from build123d import *

# Parameters (mm, degrees)
SKETCH1_W                      = 53
SKETCH1_H                      = 25
SKETCH1_R                      = 4.5
SKETCH1_R_2                    = 1.5
BASE_FLANGE1_DEPTH             = 1
EDGE_FLANGE1_STRIP_W           = 5.4732
EDGE_FLANGE1_STRIP_H           = 1
EDGE_FLANGE1_STRIP_CUT_DEPTH   = 25
EDGE_FLANGE1_STRIP_2_W         = 5.4732
EDGE_FLANGE1_STRIP_2_H         = 1
EDGE_FLANGE1_STRIP_CUT_2_DEPTH = 25
EDGE_FLANGE1_DEPTH             = 25
EDGE_FLANGE1_BEND_DEPTH        = 25
CUT_EXTRUDE1_DEPTH             = 73.584433593
CUT_EXTRUDE1_DEPTH_BACK        = 73.584433593
SKETCH13_R                     = 4.5
SKETCH13_R_2                   = 2
SKETCH13_R_3                   = 1.5
FILLET1_R                      = 12.5


# Sheet-metal steps are written as plain solids
with BuildPart() as part:
    # Sketch1 → Base-Flange1 (new body)
    with BuildSketch(Plane(origin=(0, 0, 0), x_dir=(1, 0, 0), z_dir=(0, 1, 0))):
        Rectangle(SKETCH1_W, SKETCH1_H)
        with Locations(Location((0, 0, 0), (0, 0, 270))):
            Circle(SKETCH1_R, mode=Mode.SUBTRACT)
        with Locations(Location((-7, 0, 0), (0, 0, 270))):
            Circle(SKETCH1_R_2, mode=Mode.SUBTRACT)
        with Locations(Location((7, 0, 0), (0, 0, 270))):
            Circle(SKETCH1_R_2, mode=Mode.SUBTRACT)
        with Locations(Location((0, 7, 0), (0, 0, 270))):
            Circle(SKETCH1_R_2, mode=Mode.SUBTRACT)
        with Locations(Location((0, -7, 0), (0, 0, 270))):
            Circle(SKETCH1_R_2, mode=Mode.SUBTRACT)
    extrude(amount=BASE_FLANGE1_DEPTH)

    # Edge-Flange1 strip (across the edge) → Edge-Flange1 strip cut (cut)
    with BuildSketch(Plane(origin=(-26.5, 1, -12.5), x_dir=(1, 0, 0), z_dir=(0, 0, 1))):
        with Locations((-2, -0.5)):
            Rectangle(EDGE_FLANGE1_STRIP_W, EDGE_FLANGE1_STRIP_H)
    extrude(amount=EDGE_FLANGE1_STRIP_CUT_DEPTH, mode=Mode.SUBTRACT)

    # Edge-Flange1 strip 2 (across the edge) → Edge-Flange1 strip cut 2 (cut)
    with BuildSketch(Plane(origin=(26.5, 1, 12.5), x_dir=(-1, 0, 0), z_dir=(0, 0, -1))):
        with Locations((-2, -0.5)):
            Rectangle(EDGE_FLANGE1_STRIP_2_W, EDGE_FLANGE1_STRIP_2_H)
    extrude(amount=EDGE_FLANGE1_STRIP_CUT_2_DEPTH, mode=Mode.SUBTRACT)

    # Edge-Flange1 section (across the edge) → Edge-Flange1 (add)
    with BuildSketch(Plane(origin=(-26.5, 1, -12.5), x_dir=(1, 0, 0), z_dir=(0, 0, 1))):
        with BuildLine():
            Line((-1, 0.7366), (-1, 65))
            Line((-1, 65), (0, 65))
            Line((0, 65), (0, 0.7366))
            ThreePointArc((0, 0.7366), (0.215745145, 0.215745145), (0.7366, 0))
            Line((0.7366, 0), (0.7366, -1))
            ThreePointArc((0.7366, -1), (-0.491361636, -0.491361636), (-1, 0.7366))
        make_face()
    extrude(amount=EDGE_FLANGE1_DEPTH)

    # Edge-Flange1 section 2 (across the edge) → Edge-Flange1 bend (add)
    with BuildSketch(Plane(origin=(26.5, 1, 12.5), x_dir=(-1, 0, 0), z_dir=(0, 0, -1))):
        with BuildLine():
            Line((-1, 0.7366), (-1, 65))
            Line((-1, 65), (0, 65))
            Line((0, 65), (0, 0.7366))
            ThreePointArc((0, 0.7366), (0.215745145, 0.215745145), (0.7366, 0))
            Line((0.7366, 0), (0.7366, -1))
            ThreePointArc((0.7366, -1), (-0.491361636, -0.491361636), (-1, 0.7366))
        make_face()
    extrude(amount=EDGE_FLANGE1_BEND_DEPTH)

    # Sketch13 → Cut-Extrude1 (cut, two sides: drawn at the far end of the back side and taken through both)
    with BuildSketch(Plane(origin=(0, 0, 0), x_dir=(0, 0, -1), z_dir=(1, 0, 0)).offset(-CUT_EXTRUDE1_DEPTH_BACK)):
        with Locations((0, 53.5)):
            Circle(SKETCH13_R)
        with Locations((-7, 53.5)):
            Circle(SKETCH13_R_2)
        with Locations((7, 53.5)):
            Circle(SKETCH13_R_2)
        with Locations((0, 46.5)):
            Circle(SKETCH13_R_2)
        with Locations((0, 60.5)):
            Circle(SKETCH13_R_2)
        with Locations((0, 33)):
            Circle(SKETCH13_R_3)
        with Locations((0, 15)):
            Circle(SKETCH13_R_3)
    extrude(amount=CUT_EXTRUDE1_DEPTH + CUT_EXTRUDE1_DEPTH_BACK, mode=Mode.SUBTRACT)

    # Fillet1
    fillet1_edges = [part.edges().sort_by_distance(p)[0] for p in [
        (-27, 66, -12.5),
        (-27, 66, 12.5),
        (27, 66, -12.5),
        (27, 66, 12.5),
    ]]
    fillet(fillet1_edges, radius=FILLET1_R - 0.0001)  # a hair under: the kernel refuses the full size


solid = part.part
The listing builds one solid part. Answer for the finished solid, in the listing's coordinates (mm). A direction names the side the tool comes from. Give positions to 0.01 mm unless a question says otherwise; leave off trailing zeros. Write each loop counter-clockwise with the first axis right and the second up, starting at its lowest first coordinate (ties: lowest second). Pieces come first, ordered by that corner, then holes.
Item 1: Determine the mould class of faces 1 (the cylindrical face through (5.536, 0.493, -0.325)), 2 (the cylindrical face through (-27.007, 44.726, -0.923)), 3 (the cylindrical face through (-26.98, 0.5, -0.18)), 4 (the cylindrical face through (-26.993, 62.241, -8.936)) for opening direction Z: released by +Z, released by -Z, zero draft, split by the parting line, or undercut.
Item 2: Section D-D, the plane z = -7.5 is taken. Write down the section's boundary in (x, y).
Item 3: Which of the six approach directions +Z, -Z, +X, -X, +Y, -Y give full straight-line access (tool end or side, diameter ignored) to faces 5 (the flat face through (-26.5, 34, 3)), 6 (the cylindrical face through (-26.993, 62.241, 8.936))?
Item 4: Section C-C, the plane x = 0 is taken. Write down the section's boundary in (y, z).
Item 5: Section B-B, the plane x = -7 is taken. Write down the section's boundary in (y, z).
Item 6: Section A-A, the plane y = 11 is taken. Write down the section's boundary in (x, z).
Item 7: Flat-ended cylindrical pins translate along their axes: P1, Ø12.5, axis at x = -1, z = 4, coming from the +Y side; P2, Ø11.5, axis at y = 53.5, z = 0, coming from the -X side. Find the tip coordinate at first contact, or state that the pin passes through.
Item 8: Find the intervals of material crossed by line 1 along Z through (x, y) = (27.25, 53.5); line 2 along X through (y, z) = (7.5, 0.75); line 3 along Y through (x, z) = (-26.75, 0), in increasing order.
Completed:
1. face 1: undercut
1. face 2: undercut
1. face 3: zero draft
1. face 4: released by -Z
2. outline: (-27.5, 1.74) arc R1.74 ccw to (-25.76, 0) - (-1.41, 0) - (-1.41, 1) - (-25.76, 1) arc R0.74 cw to (-26.5, 1.74) - (-26.5, 51.56) - (-27.5, 51.56) - close; (-27.5, 55.44) - (-26.5, 55.44) - (-26.5, 63.5) - (-27.5, 63.5) - close; (1.41, 0) - (25.76, 0) arc R1.74 ccw to (27.5, 1.74) - (27.5, 51.56) - (26.5, 51.56) - (26.5, 1.74) arc R0.74 cw to (25.76, 1) - (1.41, 1) - close; (26.5, 55.44) - (27.5, 55.44) - (27.5, 63.5) - (26.5, 63.5) - close
3. face 5: +Z, -Z, +Y
3. face 6: +Z, +X, -X, +Y
4. outline: (0, -12.5) - (1, -12.5) - (1, -8.5) - (0, -8.5) - close; (0, -5.5) - (1, -5.5) - (1, -4.5) - (0, -4.5) - close; (0, 4.5) - (1, 4.5) - (1, 5.5) - (0, 5.5) - close; (0, 8.5) - (1, 8.5) - (1, 12.5) - (0, 12.5) - close
5. outline: (0, -12.5) - (1, -12.5) - (1, -1.5) - (0, -1.5) - close; (0, 1.5) - (1, 1.5) - (1, 12.5) - (0, 12.5) - close
6. outline: (-27.5, -12.5) - (-26.5, -12.5) - (-26.5, 12.5) - (-27.5, 12.5) - close; (26.5, -12.5) - (27.5, -12.5) - (27.5, 12.5) - (26.5, 12.5) - close
7. P1: stops at y = 1
7. P2: stops at x = -27.5
8. line 1: z = -12.5 to -9, -5 to -4.5, 4.5 to 5, 9 to 12.5
8. line 2: x = -27.5 to -26.5, 26.5 to 27.5
8. line 3: y = 0.31 to 13.5, 16.5 to 31.5, 34.5 to 44.5, 48.5 to 49, 58 to 58.5, 62.5 to 66
